Can you work these out from the model? Positions are in its coordinate system, mm. Face numbers are marked on the shaded views. A direction names the side the tool comes from. Coordinates: 2 decimals unless noted, no trailing zeros. Write each loop counter-clockwise with the first axis right and the second up, starting at its lowest first coordinate (ties: lowest second). Pieces come first, ordered by that corner, then holes.
```python
from build123d import *

# Parameters (mm, degrees)
SKETCH_1_R          = 11
EXTRUDE_1_DEPTH     = 3.2
SKETCH_2_R          = 5
EXTRUDE_2_DEPTH     = 10
SKETCH_3_R          = 4
CUT_EXTRUDE_1_DEPTH = 15
SKETCH_4_R          = 1.75
CUT_EXTRUDE_2_DEPTH = 7
CUT_EXTRUDE_4_DEPTH = 19.493242009
SKETCH_7_R          = 5
SKETCH_7_R_2        = 4
EXTRUDE_3_DEPTH     = 1.5


with BuildPart() as part:
    # 草图1 → 凸台-拉伸1 (new body)
    with BuildSketch(Plane.XY):
        Circle(SKETCH_1_R)
    extrude(amount=EXTRUDE_1_DEPTH)

    # 草图2 → 凸台-拉伸2 (add)
    with BuildSketch(Plane.XY.offset(3.2)):
        Circle(SKETCH_2_R)
    extrude(amount=EXTRUDE_2_DEPTH)

    # 草图3 → 切除-拉伸1 (cut)
    with BuildSketch(Plane.XY.offset(13.2)):
        Circle(SKETCH_3_R)
    extrude(amount=-CUT_EXTRUDE_1_DEPTH, mode=Mode.SUBTRACT)

    # 草图4 → 切除-拉伸2 (cut)
    with BuildSketch(Plane(origin=(0, 0, 0), x_dir=(-1, 0, 0), z_dir=(0, 0, -1))):
        with Locations((0, 8)):
            Circle(SKETCH_4_R)
        with Locations((0, -8)):
            Circle(SKETCH_4_R)
    extrude(amount=-CUT_EXTRUDE_2_DEPTH, mode=Mode.SUBTRACT)

    # 草图6 → 切除-拉伸4 (cut, through all)
    with BuildSketch(Plane.XY.offset(3.2)):
        Polygon((-5, 0), (-5, 10.334769888), (-11, 10.334769888), (-11, -9.812151942), (-5, -9.812151942), align=None)
        Polygon((11, -9.812151942), (5, -9.812151942), (5, 0), (5, 10.334769888), (11, 10.334769888), align=None)
    extrude(amount=-CUT_EXTRUDE_4_DEPTH, mode=Mode.SUBTRACT)

    # 草图7 → 凸台-拉伸3 (add)
    with BuildSketch(Plane(origin=(0, 0, 0), x_dir=(-1, 0, 0), z_dir=(0, 0, -1))):
        with Locations(Location((0, 0, 0), (0, 0, 180))):
            Circle(SKETCH_7_R)
        with Locations(Location((0, 0, 0), (0, 0, 180))):
            Circle(SKETCH_7_R_2, mode=Mode.SUBTRACT)
    extrude(amount=EXTRUDE_3_DEPTH)


solid = part.part
```
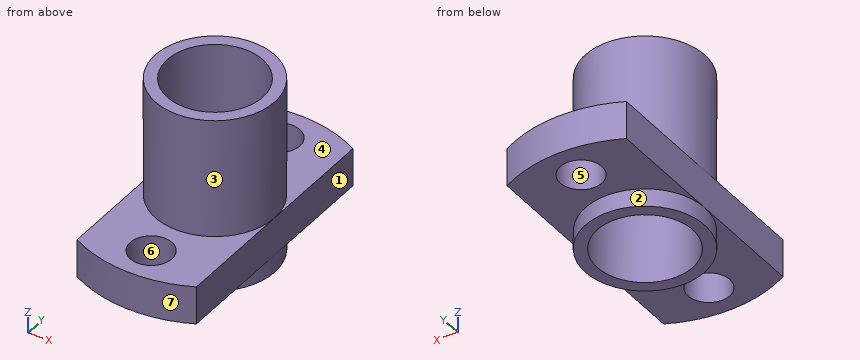
1. If we section it at C-C, the plane y = -8: List the corners of the cut face in (x, z) for me.
2. I'm going to push flat-ended pins straight in: P1, Ø2, axis at x = 0, y = 8, coming from the +Z side; P2, Ø5, axis at x = 1.5, y = 8, coming from the +Z side; P3, Ø4, axis at y = -3, z = 5.5, coming from the -X side; P4, Ø1, axis at y = 5, z = 10.5, coming from the -X side. Where does each tip first touch, or does it pass through?
3. If we section it at D-D, the plane x = -3.5: List the corners of the cut face in (y, z) for me, plus the area to 3 significant figures.
4. If we section it at A-A, the plane z = 2.5: List the corners of the cut face in (x, y) for me, plus the area to 3 significant figures.
5. We'd pull the mould along X, two halves only. Please class the marked faces 4, 5, 6 and 7: released by +X, released by -X, zero draft, split by the parting line, or undercut.
6. If we section it at B-B, the plane x = 0: List the corners of the cut face in (y, z) for me, plus the area to 3 significant figures.
7. If I drill on L1, parallel to Y at x = 0, z = 2.35; L2, parallel to Y at x = 1, z = 1.25; L3, parallel to Z at x = -3.75, y = -4.25, over which ranges is the centre line in solid material (lowest first)?
8. Which directions (+Z, -Z, +X, -X, +Y, -Y) give clear straight access to the entire face, cutting with the end or side of a thin tool? Please do the marked faces 1, 2 and 3.
Answers:
1. outline: (-5, 0) - (-1.75, 0) - (-1.75, 3.2) - (-5, 3.2) - close; (1.75, 0) - (5, 0) - (5, 3.2) - (1.75, 3.2) - close
2. P1: passes through
2. P2: stops at z = 3.2
2. P3: stops at x = -4.9
2. P4: stops at x = -2.18
3. outline: (-10.43, 0) - (-3.57, 0) - (-3.57, -1.5) - (-1.94, -1.5) - (-1.94, 13.2) - (-3.57, 13.2) - (-3.57, 3.2) - (-10.43, 3.2) - close; (1.94, -1.5) - (3.57, -1.5) - (3.57, 0) - (10.43, 0) - (10.43, 3.2) - (3.57, 3.2) - (3.57, 13.2) - (1.94, 13.2) - close
3. area: 91.9 mm2
4. outline: (-5, -9.8) arc R11 ccw to (5, -9.8) - (5, 9.8) arc R11 ccw to (-5, 9.8) - close; hole circle Ø8 at (0, 0); hole circle Ø3.5 at (0, -8); hole circle Ø3.5 at (0, 8)
4. area: 143 mm2
5. face 4: zero draft
5. face 5: undercut
5. face 6: undercut
5. face 7: split by the parting line
6. outline: (-11, 0) - (-9.75, 0) - (-9.75, 3.2) - (-11, 3.2) - close; (-6.25, 0) - (-5, 0) - (-5, -1.5) - (-4, -1.5) - (-4, 13.2) - (-5, 13.2) - (-5, 3.2) - (-6.25, 3.2) - close; (4, -1.5) - (5, -1.5) - (5, 0) - (6.25, 0) - (6.25, 3.2) - (5, 3.2) - (5, 13.2) - (4, 13.2) - close; (9.75, 0) - (11, 0) - (11, 3.2) - (9.75, 3.2) - close
6. area: 45.4 mm2
7. L1: y = -11 to -9.75, -6.25 to -4, 4 to 6.25, 9.75 to 11
7. L2: y = -10.95 to -9.44, -6.56 to -3.87, 3.87 to 6.56, 9.44 to 10.95
7. L3: z = 0 to 3.2
8. face 1: +Z, -Z, +X, +Y, -Y
8. face 2: -Z
8. face 3: +Z
